Here's how the part is built. I have some questions about the finished solid (model axes, mm). Round coordinates to 2 decimals unless told otherwise and drop trailing zeros. Write item = value, one per line. Start each with the question number.
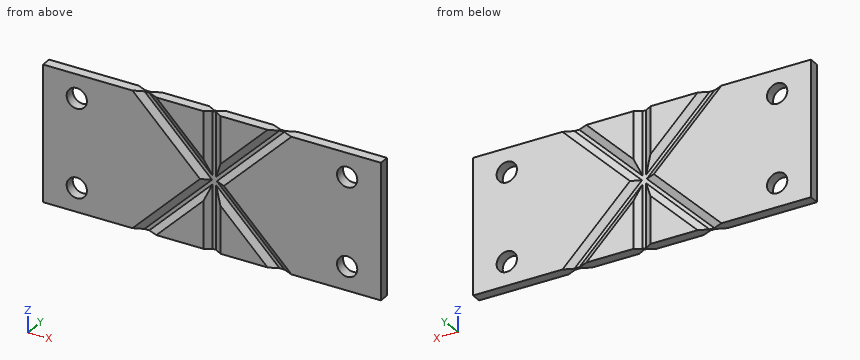
Autodesk Inventor part; units mm, degrees
ref_plane "YZ Plane" through (0, 0, 0) normal (1, 0, 0) x (0, 1, 0)
ref_plane "XZ Plane" through (0, 0, 0) normal (0, 1, 0) x (-1, 0, 0)
ref_plane "XY Plane" through (0, 0, 0) normal (0, 0, 1) x (1, 0, 0)
sketch "Sketch1" plane through (0, 0, 0) normal (0, 1, 0) x (-1, 0, 0)
  line L0 (0, 0) -> (50, 0)
  line L1 (50, 0) -> (50, -20)
  line L2 (50, -20) -> (0, -20)
  line L3 (0, -20) -> (0, 0)
  line L4 (25, 0) -> (25, -20)
  line L5 (25, -20) -> (35, -20)
  line L6 (25, 0) -> (35, 0)
  line L7 (25, 0) -> (15, 0)
  line L8 (25, -20) -> (15, -20)
  line L9 (15, -20) -> (25, -10)
  line L10 (25, -10) -> (15, 0)
  line L11 (25, -10) -> (35, -20)
  line L12 (25, -10) -> (35, 0)
  line L13 (25.25, 2.5) -> (24.75, 2.5)
  line L14 (24.75, 2.5) -> (24.75, -22.5)
  line L15 (24.75, -22.5) -> (25.25, -22.5)
  line L16 (25.25, -22.5) -> (25.25, 2.5)
  line L17 (25.25, 2.5) -> (24.75, -22.5) construction
  line L18 (24.75, 2.5) -> (25.25, -22.5) construction
  line L19 (7.4991, 7.8544) -> (7.1456, 7.5009)
  line L20 (7.1456, 7.5009) -> (42.5009, -27.8544)
  line L21 (42.5009, -27.8544) -> (42.8544, -27.5009)
  line L22 (42.8544, -27.5009) -> (7.4991, 7.8544)
  line L23 (7.4991, 7.8544) -> (42.5009, -27.8544) construction
  line L24 (7.1456, 7.5009) -> (42.8544, -27.5009) construction
  line L25 (42.8544, 7.5009) -> (42.5009, 7.8544)
  line L26 (42.5009, 7.8544) -> (7.1456, -27.5009)
  line L27 (7.1456, -27.5009) -> (7.4991, -27.8544)
  line L28 (7.4991, -27.8544) -> (42.8544, 7.5009)
  line L29 (42.8544, 7.5009) -> (7.1456, -27.5009) construction
  line L30 (42.5009, 7.8544) -> (7.4991, -27.8544) construction
  point P0 (14.6464, -20)
  point P1 (24.6464, -10)
  point P2 (14.6464, 0)
  point P3 (24.75, -10.6036)
  point P4 (15.3536, -20)
  point P5 (24.75, -20)
  point P6 (34.6464, -20)
  point P7 (25.25, -10.6036)
  point P8 (25.25, -20)
  point P9 (15.3536, 0)
  point P10 (24.75, -9.3964)
  point P11 (24.75, 0)
  point P12 (25.25, -9.3964)
  point P13 (34.6464, 0)
  point P14 (25.25, 0)
  point P15 (35.3536, 0)
  point P16 (25.3536, -10)
  point P17 (35.3536, -20)
  dimension "d0" = 50
  dimension "d1" = 20
  dimension "d2" = 10
  dimension "d3" = 10
  dimension "d4" = 10
  dimension "d5" = 10
  dimension "d6" = 0.5
  dimension "d7" = 25
  dimension "d8" = 0.5
  dimension "d9" = 50
  dimension "d10" = 0.5
  dimension "d11" = 50
extrude "Extrusion1" add sketch "Sketch1" along normal blind 1.5 contours L0 L20 L26 L2 L3 | L0 L14 L22 | L28 L14 L2 | L0 L26 L16 | L20 L2 L16 | L28 L0 L1 L2 L22
ref_plane "Work Plane1" through (0, 0.75, 0) normal (0, 1, 0) x (1, 0, 0)
sketch "Sketch2" plane through (0, 0.75, 0) normal (0, 1, 0) x (1, 0, 0)
  line L0 (-50, 20) -> (-50, 0)
  line L1 (-35.3536, 20) -> (-50, 20)
  line L2 (-25.3536, 10) -> (-35.3536, 20)
  line L3 (-35.3536, 0) -> (-25.3536, 10)
  line L4 (-50, 0) -> (-35.3536, 0)
  line L5 (-25.25, 9.3964) -> (-34.6464, 0)
  line L6 (-25.25, 0) -> (-25.25, 9.3964)
  line L7 (-34.6464, 0) -> (-25.25, 0)
  line L8 (-24.75, 9.3964) -> (-24.75, 0)
  line L9 (-15.3536, 0) -> (-24.75, 9.3964)
  line L10 (-24.75, 0) -> (-15.3536, 0)
  line L11 (-24.6464, 10) -> (-14.6464, 0)
  line L12 (-14.6464, 20) -> (-24.6464, 10)
  line L13 (0, 20) -> (-14.6464, 20)
  line L14 (0, 0) -> (0, 20)
  line L15 (-14.6464, 0) -> (0, 0)
  line L16 (-15.3536, 20) -> (-24.75, 20)
  line L17 (-24.75, 10.6036) -> (-15.3536, 20)
  line L18 (-24.75, 20) -> (-24.75, 10.6036)
  line L19 (-25.25, 20) -> (-34.6464, 20)
  line L20 (-25.25, 10.6036) -> (-25.25, 20)
  line L21 (-34.6464, 20) -> (-25.25, 10.6036)
  line L22 (-50, 0) -> (-35.3536, 0)
  line L23 (-50, 0) -> (0, 0)
  line L24 (-50, 20) -> (0, 20)
extrude "Extrusion2" add sketch "Sketch2" along normal mid plane 0.29 contours L24 L21 L20 L18 L17 L12 L11 L23 L9 L8 L6 L5 L3 L2
chamfer "Chamfer1" distance 1 distance2 0.605 1 edges at (-30.3536, 1.5, -5) measured on face at (-40.2357, 1.5, -13.3333)
chamfer "Chamfer2" distance 1 distance2 0.605 1 edges at (-29.9482, 1.5, -4.6982) measured on face at (-28.3821, 1.5, -3.1321)
chamfer "Chamfer3" distance 1 distance2 0.605 1 edges at (-30.7069, 1.5, -15.3534) measured on face at (-40.7069, 1.5, -13.3333)
chamfer "Chamfer4" distance 1 distance2 0.605 1 edges at (-29.9482, 1.5, -15.3018) measured on face at (-28.3821, 1.5, -16.8679)
chamfer "Chamfer5" distance 1 distance2 0.605 1 edges at (-25.25, 1.5, -16.0085) measured on face at (-27.911, 1.5, -17.339)
chamfer "Chamfer6" distance 1 distance2 0.605 1 edges at (-24.75, 1.5, -15.3018) measured on face at (-21.6179, 1.5, -16.8679)
chamfer "Chamfer7" distance 1 distance2 0.605 1 edges at (-25.25, 1.5, -3.9915) measured on face at (-27.911, 1.5, -2.661)
chamfer "Chamfer8" distance 1 distance2 0.605 1 edges at (-24.75, 1.5, -4.6982) measured on face at (-21.6179, 1.5, -3.1321)
chamfer "Chamfer9" distance 1 distance2 0.605 1 edges at (-19.552, 1.5, -4.1985) measured on face at (-20.9515, 1.5, -2.799)
chamfer "Chamfer10" distance 1 distance2 0.605 1 edges at (-19.6464, 1.5, -5) measured on face at (-9.7643, 1.5, -6.6667)
chamfer "Chamfer11" distance 1 distance2 0.605 1 edges at (-19.552, 1.5, -15.8015) measured on face at (-20.9515, 1.5, -17.201)
chamfer "Chamfer12" distance 1 distance2 0.605 1 edges at (-19.2931, 1.5, -15.3534) measured on face at (-9.2931, 1.5, -13.3333)
chamfer "Chamfer13" distance 0.605 distance2 1 1 edges at (-29.9482, 0, -15.3018) measured on face at (-31.5143, 0.2017, -16.8679)
chamfer "Chamfer14" distance 0.605 distance2 1 1 edges at (-30.3536, 0, -15) measured on face at (-28.6869, 0.2017, -13.3333)
chamfer "Chamfer15" distance 0.605 distance2 1 1 edges at (-25.25, 0, -16.0085) measured on face at (-25.25, 0.4033, -14.2069)
chamfer "Chamfer16" distance 0.605 distance2 1 1 edges at (-24.75, 0, -15.3018) measured on face at (-24.75, 0.2017, -16.8679)
chamfer "Chamfer17" distance 0.605 distance2 1 1 edges at (-19.552, 0, -15.8015) measured on face at (-21.2847, 0.4033, -14.0689)
chamfer "Chamfer18" distance 0.605 distance2 1 1 edges at (-19.6464, 0, -15) measured on face at (-17.9798, 0.2017, -16.6667)
chamfer "Chamfer19" distance 0.605 distance2 1 1 edges at (-19.2931, 0, -4.6466) measured on face at (-21.0775, 0.4033, -6.4311)
chamfer "Chamfer20" distance 0.605 distance2 1 1 edges at (-20.0518, 0, -4.6982) measured on face at (-18.4857, 0.2017, -3.1321)
chamfer "Chamfer21" distance 0.605 distance2 1 1 edges at (-24.75, 0, -3.9915) measured on face at (-24.75, 0.4033, -5.7931)
chamfer "Chamfer22" distance 0.605 distance2 1 1 edges at (-25.25, 0, -4.6982) measured on face at (-25.25, 0.2017, -3.1321)
chamfer "Chamfer23" distance 0.605 distance2 1 1 edges at (-30.448, 0, -4.1985) measured on face at (-28.7153, 0.4033, -5.9311)
chamfer "Chamfer24" distance 0.605 distance2 1 1 edges at (-30.7069, 0, -4.6466) measured on face at (-28.9225, 0.4033, -6.4311)
sketch "Sketch3" plane through (0, 1.5, 0) normal (0, 1, 0) x (1, 0, 0)
  line L0 (-36.7678, 20) -> (-26.7678, 10)
  line L1 (-36.7678, 20) -> (-50, 20)
  line L2 (-50, 20) -> (-50, 0)
  line L3 (-50, 0) -> (-36.7678, 0)
  line L4 (-26.7678, 10) -> (-36.7678, 0)
  line L5 (-23.2322, 10) -> (-13.2322, 20)
  line L6 (-13.2322, 0) -> (-23.2322, 10)
  line L7 (-13.2322, 0) -> (0, 0)
  line L8 (0, 0) -> (0, 20)
  line L9 (0, 20) -> (-13.2322, 20)
  line L10 (-26.7678, 10) -> (-23.2322, 10)
  line L11 (-45, 16.5) -> (-45, 3.5)
  line L12 (-45, 3.5) -> (-5, 3.5)
  line L13 (-5, 3.5) -> (-5, 16.5)
  line L14 (-5, 16.5) -> (-45, 16.5)
  line L15 (-45, 16.5) -> (-5, 3.5) construction
  line L16 (-45, 3.5) -> (-5, 16.5) construction
  line L17 (-50, 0) -> (-36.7678, 0)
  circle A0 centre (-45, 16.5) radius 1.5
  circle A1 centre (-45, 3.5) radius 1.5
  circle A2 centre (-5, 16.5) radius 1.5
  circle A3 centre (-5, 3.5) radius 1.5
  point P0 (-25, 10)
  dimension "d88" = 13
  dimension "d89" = 40
  dimension "d90" = 3
  dimension "d91" = 3
  dimension "d92" = 3
  dimension "d93" = 3
extrude "Extrusion3" cut sketch "Sketch3" against normal blind 4 contours A0 L11 L14 | L14 L11 A0 | A2 L13 L14 | L14 L13 A2 | A1 L11 L12 | L12 L11 A1 | A3 L13 L12 | L12 L13 A3
properties part number "test_hangle_org_2"
Item 1: I want a section at A-A, the plane y = 1.15. State how many separate pieces and enclosed holes the cut face has, then the cut area to 3 significant figures.
Item 2: Please list where these lines run through material, in increasing order: line 1 (Z direction, x = -5, y = 0.6); line 2 (X direction, y = 0.85, z = -3.5); line 3 (Z direction, x = -6, y = 0.9). Write a range as [from, to].
Item 3: Will this pin go through, and if not, where does the flat tip stop? pin 1 Ø5 at (x, z) = (-45, -3.5) entering from -Y.
Worked out:
q1.separate_pieces = 6
q1.enclosed_holes = 4
q1.area = 874 mm2
q2.line_1 = [-20, -18], [-15, -5], [-2, 0]
q2.line_2 = [-50, -46.5], [-43.5, -6.5], [-3.5, 0]
q2.line_3 = [-20, -17.62], [-15.38, -4.62], [-2.38, 0]
q3.pin_1 = 0
